Can you work these out from the model? Positions are in its coordinate system, mm. A direction names the side the tool comes from. Give positions to 0.01 mm unless a question says otherwise; leave off trailing zeros. Order: outer loops, then holes, each group sorted by start corner. A loop starts at its lowest first (then second) coordinate and runs counter-clockwise, first axis right, second up. Notation, with made-up numbers: (4.25, -11) - (34.25, -11) arc R20 cw to (34.25, 5) - close; hole circle Ø1 at (47, -21.5). An arc over 180 degrees is marked (long way). Answer as a JSON object with one key per item and string values.
```python
from build123d import *

# Parameters (mm, degrees)
PAD_DEPTH    = 10
SKETCH001_R  = 33.5
POCKET_DEPTH = 5


with BuildPart() as part:
    # Sketch → Pad (new body)
    with BuildSketch(Plane.XY):
        Polygon((0, -28.5), (20, -28.5), (20, 0), (117, 0), (117, -28.5), (137, -28.5), (137, -58.5), (117, -58.5), (117, -87), (20, -87), (20, -58.5), (0, -58.5), align=None)
    extrude(amount=-PAD_DEPTH)

    # Sketch001 → Pocket (cut)
    with BuildSketch(Plane.XY):
        with Locations((73.5, -43.5)):
            Circle(SKETCH001_R)
    extrude(amount=-POCKET_DEPTH, mode=Mode.SUBTRACT)


solid = part.part
```
Q1. I need wall thicknesses on L1, parallel to Y at x = 73.5, z = -3.05; L2, parallel to X at y = -16, z = -8.5; L3, parallel to Z at x = 76, y = -35.5. Which ranges of each line are inside material? Lowest first, please.
Recorded:
{"L1": "y = -87 to -77, -10 to 0", "L2": "x = 20 to 117", "L3": "z = -10 to -5"}
Q2. If we section it at A-A, the plane z = -7: Please give me the cut outline in (x, y), then the cut area to 3 significant figures.
Recorded:
{"outline": "(0, -58.5) - (20, -58.5) - (20, -87) - (117, -87) - (117, -58.5) - (137, -58.5) - (137, -28.5) - (117, -28.5) - (117, 0) - (20, 0) - (20, -28.5) - (0, -28.5) - close", "area": "9,640 mm^2"}
Q3. If we section it at C-C, the plane y = -40: Please give me the cut outline in (x, z).
Recorded:
{"outline": "(0, -10) - (137, -10) - (137, 0) - (106.82, 0) - (106.82, -5) - (40.18, -5) - (40.18, 0) - (0, 0) - close"}
Q4. Which directions (+Z, -Z, +X, -X, +Y, -Y) give clear straight access to the entire face, cutting with the end or side of a thin tool? Please do faces 5 (the face through (10, -58.5, -5)), 6 (the face through (117, -73, -5)), 7 (the face through (127, -28.5, -5)), 8 (the face through (10, -28.5, -5)).
Recorded:
{"face 5": "+Z, -Z, -X, -Y", "face 6": "+Z, -Z, +X, -Y", "face 7": "+Z, -Z, +X, +Y", "face 8": "+Z, -Z, -X, +Y"}
Q5. We'd pull the mould along Y, two halves only. Please class faces 1 (the face through (66.238, -76.203, -2.465)), 2 (the face through (20, -73, -5)), 3 (the face through (69, -87, -5)), 4 (the face through (73, -43, -5)): released by +Y, released by -Y, zero draft, split by the parting line, or undercut.
Recorded:
{"face 1": "undercut", "face 2": "zero draft", "face 3": "released by -Y", "face 4": "undercut"}
Q6. If we section it at B-B, the plane x = 73.5: Please give me the cut outline in (y, z), then the cut area to 3 significant figures.
Recorded:
{"outline": "(-87, -10) - (0, -10) - (0, 0) - (-10, 0) - (-10, -5) - (-77, -5) - (-77, 0) - (-87, 0) - close", "area": "535 mm^2"}
Q7. I'm going to push flat-ended pins straight in: pin 1 Ø5 at (y, z) = (-73.5, -6) entering from -X; pin 2 Ø3 at (x, z) = (100, -1.5) entering from +Y; pin 3 Ø5 at (x, z) = (128, -2.5) entering from -Y; pin 4 Ø3 at (x, z) = (7, -4) entering from +Y. Where does each tip first touch, or does it pass through?
Recorded:
{"pin 1": "stops at x = 20", "pin 2": "stops at y = 0", "pin 3": "stops at y = -58.5", "pin 4": "stops at y = -28.5"}
